Design review of the part built by this model. Coordinates are the model's own, in mm. Face numbers are marked on the shaded views. A direction names the side the tool comes from. Coordinates: 2 decimals unless noted, no trailing zeros. Loops run counter-clockwise (first coordinate to the right, second up) from the corner with the lowest first, then second, coordinate; pieces in that order, holes last. Notation, with made-up numbers: (37.25, -28.75) -> (96.25, -28.75) arc R27 cw to (96.25, 7.25) -> close; hole circle Ø2 at (5, 51). An arc over 180 degrees is marked (long way). Use CSV: the item, a comma, the result in double quotes.
```python
from build123d import *

# Parameters (mm, degrees)
SKETCH2_W           = 35
SKETCH2_H           = 10
BOSS_EXTRUDE1_DEPTH = 4
CUT_EXTRUDE1_DEPTH  = 4
SKETCH4_W           = 6.2
SKETCH4_H           = 1.5
CUT_EXTRUDE2_DEPTH  = 4.4
SKETCH5_W           = 6.2
SKETCH5_H           = 1.4
CUT_EXTRUDE3_DEPTH  = 4.4
FILLET1_R           = 1
FILLET2_R           = 1
CHAMFER1_SIZE       = 0.5


with BuildPart() as part:
    # Sketch2 → Boss-Extrude1 (new body)
    with BuildSketch(Plane(origin=(0, 0, 0), x_dir=(1, 0, 0), z_dir=(0, 1, 0))):
        Rectangle(SKETCH2_W, SKETCH2_H)
    extrude(amount=BOSS_EXTRUDE1_DEPTH)

    # Sketch3 → Cut-Extrude1 (cut)
    with BuildSketch(Plane(origin=(0, 4, 0), x_dir=(1, 0, 0), z_dir=(0, 1, 0))):
        with BuildLine():
            Line((-11.3, 0.932737905), (-11.3, 3.2))
            Line((-11.3, 3.2), (-13.1, 3.2))
            Line((-13.1, 3.2), (-13.1, -3.2))
            Line((-13.1, -3.2), (-11.3, -3.2))
            Line((-11.3, -3.2), (-11.3, -0.932737905))
            ThreePointArc((-11.3, -0.932737905), (-8.4, 0), (-11.3, 0.932737905))
        make_face()
        with BuildLine():
            Line((11.3, -3.2), (11.3, -0.932737905))
            ThreePointArc((11.3, -0.932737905), (8.4, 0), (11.3, 0.932737905))
            Line((11.3, 0.932737905), (11.3, 3.2))
            Line((11.3, 3.2), (13.1, 3.2))
            Line((13.1, 3.2), (13.1, -3.2))
            Line((13.1, -3.2), (11.3, -3.2))
        make_face()
    extrude(amount=-CUT_EXTRUDE1_DEPTH, mode=Mode.SUBTRACT)

    # Sketch4 → Cut-Extrude2 (cut)
    with BuildSketch(Plane.ZY.offset(17.5)):
        with Locations((0, 0.75)):
            Rectangle(SKETCH4_W, SKETCH4_H)
    extrude(amount=-CUT_EXTRUDE2_DEPTH, mode=Mode.SUBTRACT)

    # Sketch5 → Cut-Extrude3 (cut)
    with BuildSketch(Plane(origin=(17.5, 0, 0), x_dir=(0, 0, -1), z_dir=(1, 0, 0))):
        with Locations((0, 0.7)):
            Rectangle(SKETCH5_W, SKETCH5_H)
    extrude(amount=-CUT_EXTRUDE3_DEPTH, mode=Mode.SUBTRACT)

    # Fillet1
    fillet1_edges = [part.edges().sort_by_distance(p)[0] for p in [
        (-13.1, 4, 0),
        (13.1, 4, 0),
        (-13.1, 1.5, 0),
        (13.1, 1.4, 0),
    ]]
    fillet(fillet1_edges, radius=FILLET1_R)

    # Fillet2
    fillet2_edges = [part.edges().sort_by_distance(p)[0] for p in [
        (-17.5, 4, 0),
        (17.5, 4, 0),
    ]]
    fillet(fillet2_edges, radius=FILLET2_R)

    # Chamfer1
    chamfer1_edges = [part.edges().sort_by_distance(p)[0] for p in [
        (0, 4, -5),
        (0, 4, 5),
        (17.5, 1.5, 5),
        (-17.5, 1.5, 5),
        (17.207106781, 3.707106781, 5),
        (-17.207106781, 3.707106781, 5),
        (-17.5, 1.5, -5),
        (17.5, 1.5, -5),
        (17.207106781, 3.707106781, -5),
        (-17.207106781, 3.707106781, -5),
    ]]
    chamfer(chamfer1_edges, length=CHAMFER1_SIZE)


solid = part.part
```
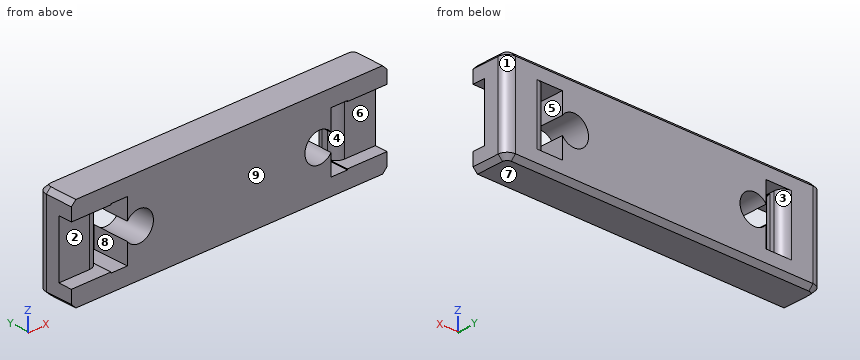
Item 1: Clearance check with flat-ended pins moving along their axes: pin 1 (1 mm diameter, centred on x = -15.5, z = 0.5, fed in from -Y); pin 2 (0.9 mm diameter, centred on y = 1, z = 1.5, fed in from -X). State where each tip first meets the part, or that it passes through.
Checked values:
pin 1,"y = 1.5"
pin 2,"x = -11.3"
Item 2: Add section C-C (z = 0). Give the boundary of the cut face in (x, y), then the cut area to 3 significant figures.
Checked values:
outline,"(-17.5, 1.5) -> (-14.1, 1.5) arc R1 ccw to (-13.1, 2.5) -> (-13.1, 3) arc R1 ccw to (-14.1, 4) -> (-16.5, 4) arc R1 ccw to (-17.5, 3) -> close; (-8.4, 0) -> (8.4, 0) -> (8.4, 4) -> (-8.4, 4) -> close; (13.1, 2.4) arc R1 ccw to (14.1, 1.4) -> (17.5, 1.4) -> (17.5, 3) arc R1 ccw to (16.5, 4) -> (14.1, 4) arc R1 ccw to (13.1, 3) -> close"
area,"88.4 mm^2"
Item 3: Add section D-D (y = 0.4). Give the boundary of the cut face in (x, z), then the cut area to 3 significant figures.
Checked values:
outline,"(-17.5, -4.5) -> (-17, -5) -> (17, -5) -> (17.5, -4.5) -> (17.5, -3.1) -> (13.1, -3.1) -> (13.1, -3.2) -> (11.3, -3.2) -> (11.3, -0.93) arc R1.6 cw (long way) to (11.3, 0.93) -> (11.3, 3.2) -> (13.1, 3.2) -> (13.1, 3.1) -> (17.5, 3.1) -> (17.5, 4.5) -> (17, 5) -> (-17, 5) -> (-17.5, 4.5) -> (-17.5, 3.1) -> (-13.1, 3.1) -> (-13.1, 3.2) -> (-11.3, 3.2) -> (-11.3, 0.93) arc R1.6 cw (long way) to (-11.3, -0.93) -> (-11.3, -3.2) -> (-13.1, -3.2) -> (-13.1, -3.1) -> (-17.5, -3.1) -> close"
area,"257 mm^2"
Item 4: Machinability: for the marked faces 1, 2, 3, 4 and 5, which of the approach directions +Z, -Z, +X, -X, +Y, -Y give a long, thin tool a straight path to every point of the face, cutting with its end or side? Answer none if there is none.
Checked values:
face 1,"+Z, -Z, +X, +Y"
face 2,"-X, -Y"
face 3,"+Y"
face 4,"-Y"
face 5,"+Y, -Y"
Item 5: To check wall thickness, follow line 1 along X through (y, z) = (3.05, 0); line 2 along Z through (x, y) = (-10, 1.85); line 3 along Z through (x, y) = (12.5, 1.8). State the ranges of each line that lie inside material, in increasing order.
Checked values:
line 1,"-17.5 to -13.1, -8.4 to 8.4, 13.1 to 17.5"
line 2,"-5 to -1.6, 1.6 to 5"
line 3,"-5 to -3.2, 3.2 to 5"
Item 6: Add section B-B (z = 2.75). Give the boundary of the cut face in (x, y), then the cut area to 3 significant figures.
Checked values:
outline,"(-17.5, 1.5) -> (-14.1, 1.5) arc R1 ccw to (-13.1, 2.5) -> (-13.1, 3) arc R1 ccw to (-14.1, 4) -> (-16.5, 4) arc R1 ccw to (-17.5, 3) -> close; (-11.3, 0) -> (11.3, 0) -> (11.3, 4) -> (-11.3, 4) -> close; (13.1, 2.4) arc R1 ccw to (14.1, 1.4) -> (17.5, 1.4) -> (17.5, 3) arc R1 ccw to (16.5, 4) -> (14.1, 4) arc R1 ccw to (13.1, 3) -> close"
area,"112 mm^2"
Item 7: Draft analysis for pull direction Z (two halves, no side actions). For the marked faces 6, 7, 8 and 9, state which applies: pulls with the +Z half, pulls with the -Z half, needs draft (parallel to the pull), parting line crosses it, or undercut.
Checked values:
face 6,"undercut"
face 7,"pulls with the -Z half"
face 8,"undercut"
face 9,"needs draft"
Item 8: Add section A-A (x = -10). Give the boundary of the cut face in (y, z).
Checked values:
outline,"(0, -5) -> (3.5, -5) -> (4, -4.5) -> (4, -1.6) -> (0, -1.6) -> close; (0, 1.6) -> (4, 1.6) -> (4, 4.5) -> (3.5, 5) -> (0, 5) -> close"
